from build123d import *

# Parameters (mm, degrees)
SKETCH1_R               = 9.525
BOSS_EXTRUDE1_DEPTH     = 7.9375
SKETCH2_R               = 1.1303
CUT_EXTRUDE1_DEPTH      = 1
CUT_EXTRUDE1_DEPTH_BACK = 20.05


with BuildPart() as part:
    # Sketch1 → Boss-Extrude1 (new body, symmetric)
    with BuildSketch(Plane(origin=(0, 0, 0), x_dir=(0, 0, -1), z_dir=(1, 0, 0))):
        Circle(SKETCH1_R)
        with BuildLine():
            Line((-3.76696164, 5.9), (3.76696164, 5.9))
            ThreePointArc((3.76696164, 5.9), (7, 0), (3.76696164, -5.9))
            Line((3.76696164, -5.9), (-3.76696164, -5.9))
            ThreePointArc((-3.76696164, -5.9), (-7, 0), (-3.76696164, 5.9))
        make_face(mode=Mode.SUBTRACT)
    extrude(amount=BOSS_EXTRUDE1_DEPTH, both=True)

    # Sketch2 → Cut-Extrude1 (cut, two sides)
    with BuildSketch(Plane(origin=(0, 9.525, 0), x_dir=(1, 0, 0), z_dir=(0, 1, 0))) as cut_extrude1_sk:
        with Locations((-3.175, 0)):
            Circle(SKETCH2_R)
        with Locations((3.175, 0)):
            Circle(SKETCH2_R)
    extrude(amount=CUT_EXTRUDE1_DEPTH, mode=Mode.SUBTRACT)
    extrude(cut_extrude1_sk.sketch, amount=-CUT_EXTRUDE1_DEPTH_BACK, mode=Mode.SUBTRACT)


solid = part.part
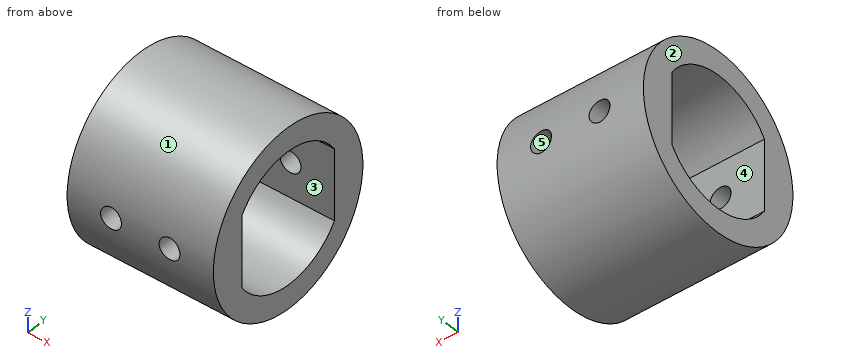
Here's how the part is built. I have some questions about the finished solid (model axes, mm). Face numbers are marked on the shaded views. A direction names the side the tool comes from. Coordinates: 2 decimals unless noted, no trailing zeros. Loops run counter-clockwise (first coordinate to the right, second up) from the corner with the lowest first, then second, coordinate; pieces in that order, holes last. Notation, with made-up numbers: (19, -37) -> (40, -37) arc R23 cw to (40, -15) -> close; hole circle Ø10 at (13.5, 32). An arc over 180 degrees is marked (long way). Use one line per item in the form item = value. Start each with the question number.
(1) We'd pull the mould along Y, two halves only. Please class the marked faces 1, 2 and 3: pulls with the +Y half, pulls with the -Y half, needs draft (parallel to the pull), parting line crosses it, or undercut.
(2) Will these pins go through, and if not, where does the flat tip stop? pin 1 (4 mm diameter, centred on x = -0.5, z = -1.5, fed in from +Y) (3 decimals); pin 2 (3 mm diameter, centred on x = 3, y = -3.5, fed in from +Z); pin 3 (1 mm diameter, centred on x = -5.5, z = 2.5, fed in from +Y); pin 4 (2.5 mm diameter, centred on x = 3.5, z = -1.5, fed in from -Y).
(3) If we section it at B-B (z = 0): Please give me the cut outline in (x, y) (1 decimal).
(4) Please list where these lines run through material, in increasing order: line 1 along X through (y, z) = (-6.9, 0); line 2 along X through (y, z) = (8, -1); line 3 along Y through (x, z) = (2.75, -1.5).
(5) If we section it at A-A (y = 0): Please give me the cut outline in (x, z) (1 decimal), then the cut area to 3 significant figures.
(6) If we section it at D-D (z = 6.25): Please give me the cut outline in (x, y), then the cut area to 3 significant figures.
(7) On a 3-axis mill with a long thin cutter (end or side, diameter ignored), from which of +Z, -Z, +X, -X, +Y, -Y can I reach the whole of each face in a straight line? I mean the marked faces 4 and 5. Say none if no direction works.
(8) If we section it at C-C (x = -3): Please give me the cut outline in (y, z) (3 decimals), then the cut area to 3 significant figures.
Verdict:
q1.face_1 = parting line crosses it
q1.face_2 = needs draft
q1.face_3 = undercut
q2.pin_1 = 9.525
q2.pin_2 = 9.31
q2.pin_3 = 9.31
q2.pin_4 = -9.51
q3.outline = (-7.9, -9.5) -> (-4.3, -9.5) -> (-4.3, -5.9) -> (-7.9, -5.9) -> close; (-7.9, 5.9) -> (-4.3, 5.9) -> (-4.3, 9.5) -> (-7.9, 9.5) -> close; (-2, -9.5) -> (2, -9.5) -> (2, -5.9) -> (-2, -5.9) -> close; (-2, 5.9) -> (2, 5.9) -> (2, 9.5) -> (-2, 9.5) -> close; (4.3, -9.5) -> (7.9, -9.5) -> (7.9, -5.9) -> (4.3, -5.9) -> close; (4.3, 5.9) -> (7.9, 5.9) -> (7.9, 9.5) -> (4.3, 9.5) -> close
q4.line_1 = -7.94 to -4.31, -2.04 to 2.04, 4.31 to 7.94
q4.line_2 = -7.94 to -3.7, -2.65 to 2.65, 3.7 to 7.94
q4.line_3 = -9.41 to -5.9, 5.9 to 9.41
q5.outline = (-7.9, -9.5) -> (7.9, -9.5) -> (7.9, -7) -> (-7.9, -7) -> close; (-7.9, 7) -> (7.9, 7) -> (7.9, 9.5) -> (-7.9, 9.5) -> close
q5.area = 80.2 mm²
q6.outline = (-7.94, -7.19) -> (7.94, -7.19) -> (7.94, -3.15) -> (-7.94, -3.15) -> close; (-7.94, 3.15) -> (7.94, 3.15) -> (7.94, 7.19) -> (-7.94, 7.19) -> close
q6.area = 128 mm²
q7.face_4 = +X, -X
q7.face_5 = +Y, -Y
q8.outline = (-9.459, -1.117) arc R9.525 ccw to (9.459, -1.117) -> (5.9, -1.117) -> (5.9, -3.767) arc R7 cw to (-5.9, -3.767) -> (-5.9, -1.117) -> close; (-9.459, 1.117) -> (-5.9, 1.117) -> (-5.9, 3.767) arc R7 cw to (5.9, 3.767) -> (5.9, 1.117) -> (9.459, 1.117) arc R9.525 ccw to start
q8.area = 126 mm²
